Model file for the job. Use its own axes, mm. Face numbers are marked on the shaded views. A direction names the side the tool comes from. Round coordinates to 2 decimals unless told otherwise and drop trailing zeros. Loops run counter-clockwise (first coordinate to the right, second up) from the corner with the lowest first, then second, coordinate; pieces in that order, holes last. Notation, with made-up numbers: M 64,-22 L 84,-22 A14 ccw 84,-14 Z; hole C 31.5,-35 d3. An arc over 180 degrees is marked long. Use a Markdown table: item, result. Add a question column.
Item 1: Tool access for the marked faces 1 and 2: list every direction of +Z, -Z, +X, -X, +Y, -Y with a clear straight run to the whole face (end or side of a thin tool).
Item 2: Saw through at B-B on y = -19.5. Write the cut outline in (x, z).
Item 3: Saw through at A-A on z = 0. Write the cut outline in (x, y).
Item 4: Wall check: L1, parallel to Y at x = -47.5, z = 10; L2, parallel to X at y = -20.5, z = 18; L3, parallel to X at y = -5, z = -5. Give the ranges that are in metal, low to high. Write a range as from..to.
Item 5: Saw through at D-D on y = -35. Write the cut outline in (x, z), then the cut area to 3 significant figures.
Item 6: Two-plate mould, pull along Z, no slides. Class the marked faces 3, 4, 5 and 6: +Z half, -Z half, draft (parallel to the pull), parting line (faces both ways), or undercut.
Item 7: Pin check, flat tips, straight feed: P1, Ø18.5, axis at x = 30.5, y = -45.5, coming from the +Z side; P2, Ø9.5, axis at x = -48.05, y = -16.07, coming from the -Z side; P3, Ø20.5, axis at x = -49, y = -54, coming from the -Z side; P4, Ø5, axis at x = 1, y = -43, coming from the +Z side. Stop position of each tip, or through.
Item 8: Saw through at C-C on x = -2.5. Write the cut outline in (y, z).
```python
from build123d import *

# Parameters (mm, degrees)
F0_R     = 12.5
F1_DEPTH = 75
F2_SIZE  = 13
F3_SIZE  = 13
F5_R     = 6
F6_DEPTH = 25
F8_R     = 12.5
F9_DEPTH = 25


with BuildPart() as f1:
    # F0 (on Front) → F1 (new body)
    with BuildSketch(Plane.XZ):
        with BuildLine():
            ThreePointArc((23.323808, -9), (20.615528, 14.142136), (0, 25))
            Line((0, 25), (-64, 25))
            Line((-64, 25), (-64, 8.888163))
            Line((-64, 8.888163), (-23.366655, 8.888163))
            ThreePointArc((-23.366655, 8.888163), (-20.581595, -14.191475), (0, -25))
            Line((0, -25), (56, -25))
            Line((56, -25), (56, 50))
            Line((56, 50), (40, 50))
            Line((40, 50), (40, -9))
            Line((40, -9), (23.323808, -9))
        make_face()
        Circle(F0_R, mode=Mode.SUBTRACT)
    extrude(amount=F1_DEPTH)

    # F2
    f2_edges = [f1.edges().sort_by_distance(p)[0] for p in [
        (48, -75, 50),
    ]]
    chamfer(f2_edges, length=F2_SIZE)

    # F3
    f3_edges = [f1.edges().sort_by_distance(p)[0] for p in [
        (48, 0, 50),
    ]]
    chamfer(f3_edges, length=F3_SIZE)

    # F5 (on face) → F6 (cut)
    with BuildSketch(Plane.XY.offset(25)):
        with Locations((-48.045456, -16.069992)):
            Circle(F5_R)
        with Locations((-48.363637, -59.024539)):
            Circle(F5_R)
    extrude(amount=-F6_DEPTH, mode=Mode.SUBTRACT)

    # F8 (on face) → F9 (cut)
    with BuildSketch(Plane.YZ.offset(56)):
        with Locations((-38.181819, 18.293647)):
            Circle(F8_R)
    extrude(amount=-F9_DEPTH, mode=Mode.SUBTRACT)


solid = f1.part
```
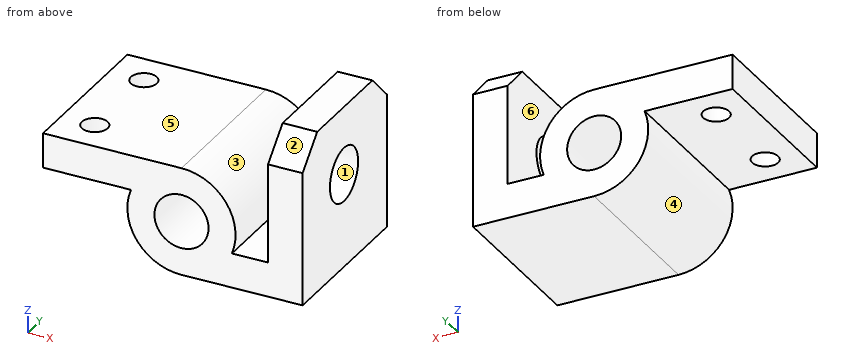
Entries:
| question | item | result |
|---|---|---|
| 1 | face 1 | +X |
| 1 | face 2 | +Z, +X, -X, -Y |
| 2 | outline | M -64,8.89 L -52.97,8.89 L -52.97,25 L -64,25 Z; M -43.12,8.89 L -23.37,8.89 A25 ccw 0,-25 L 56,-25 L 56,50 L 40,50 L 40,-9 L 23.32,-9 A25 ccw 0,25 L -43.12,25 Z; hole C 0,0 d25 |
| 3 | outline | M -25,-75 L -12.5,-75 L -12.5,0 L -25,0 Z; M 12.5,-75 L 25,-75 L 25,0 L 12.5,0 Z; M 40,-75 L 56,-75 L 56,0 L 40,0 Z |
| 4 | L1 | -75..-64.96, -53.09..-22.05, -10.09..0 |
| 4 | L2 | -64..-52.09, -44..17.35, 40..56 |
| 4 | L3 | -24.49..-11.46, 11.46..24.49, 40..56 |
| 5 | outline | M -64,8.89 L -23.37,8.89 A25 ccw 0,-25 L 56,-25 L 56,6.21 L 40,6.21 L 40,-9 L 23.32,-9 A25 ccw 0,25 L -64,25 Z; M 40,30.38 L 56,30.38 L 56,50 L 40,50 Z; hole C 0,0 d25 |
| 5 | area | 3,410 mm2 |
| 6 | face 3 | undercut |
| 6 | face 4 | undercut |
| 6 | face 5 | +Z half |
| 6 | face 6 | draft |
| 7 | P1 | z = 13.17 |
| 7 | P2 | through |
| 7 | P3 | z = 8.89 |
| 7 | P4 | z = 25 |
| 8 | outline | M -75,-24.87 L 0,-24.87 L 0,-12.25 L -75,-12.25 Z; M -75,12.25 L 0,12.25 L 0,25 L -75,25 Z |
